Check sheet for the modelled part. Datum: model origin and axes. Units: mm. Coordinates: 2 decimals unless noted, no trailing zeros. Loops run counter-clockwise (first coordinate to the right, second up) from the corner with the lowest first, then second, coordinate; pieces in that order, holes last. Notation, with made-up numbers: (-29.5, -35.5) - (26.5, -35.5) arc R33 cw to (26.5, -3.5) - close; hole circle Ø11 at (-17.5, 81). An arc over 180 degrees is marked (long way). Write each question's results on one line, items separated by ' | '. Start each with the question number.
1. Gauge pin test, flat end, axial feed: P1, Ø1, axis at x = -3, z = 1.5, coming from the +Y side. Record the tip position at first contact, or that the pin passes through.
2. Cross-section at A-A (x = 21). Record the cut outline in (y, z).
3. Cross-section at B-B (y = 1). Record the cut outline in (x, z), and give its area (4 significant figures).
4. Cross-section at C-C (z = 1.85). Record the cut outline in (x, y).
5. Cross-section at D-D (x = -19). Record the cut outline in (y, z).
6. Draft check along Y on faces 1 (the face through (0.28, -22.22, 1.27)), 2 (the face through (24.05, -20.26, 1.27)), 3 (the face through (29, -19, 1)), 4 (the face through (10, 10, 1)). Enter one of: released by +Y, released by -Y, zero draft, split by the parting line, or undercut.
7. Thickness scan on line 1 (Y direction, x = -19, z = 1.3); line 2 (X direction, y = -20.5, z = 1.35); line 3 (Y direction, x = -22, z = 0.1). Record the ranges inside material, lowest first. Write a range as [from, to].
```python
from build123d import *

# Parameters (mm, degrees)
BOSS_EXTRUDE1_DEPTH = 2.5
SKETCH2_R           = 3.3
CUT_EXTRUDE1_DEPTH  = 3.5
LPATTERN1_COUNT     = 3
LPATTERN1_PITCH     = 20
LPATTERN2_COUNT     = 3
LPATTERN2_PITCH     = 20


with BuildPart() as part:
    # Sketch1 → Boss-Extrude1 (new body)
    with BuildSketch(Plane.XY):
        Polygon((-9, 29), (29, -9), (29, -29), (-29, -29), (-29, 29), align=None)
    extrude(amount=BOSS_EXTRUDE1_DEPTH)

    # Sketch2 → Cut-Extrude1 (cut, through all)
    with BuildSketch(Plane.XY.offset(2.5)):
        with Locations((-19, -19)):
            Circle(SKETCH2_R)
    cut_extrude1 = extrude(amount=-CUT_EXTRUDE1_DEPTH, mode=Mode.SUBTRACT)

    # LPattern1: Cut-Extrude1 ×3
    with Locations(*[(i * LPATTERN1_PITCH, 0, 0) for i in range(1, LPATTERN1_COUNT)]):
        add(cut_extrude1, mode=Mode.SUBTRACT)

    # LPattern2: Cut-Extrude1 ×3
    with Locations(*[(0, i * LPATTERN2_PITCH, 0) for i in range(1, LPATTERN2_COUNT)]):
        add(cut_extrude1, mode=Mode.SUBTRACT)


solid = part.part
```
Established:
1) P1: y = 23.5
2) outline: (-29, 0) - (-22.3, 0) - (-22.3, 2.5) - (-29, 2.5) - close; (-15.7, 0) - (-1, 0) - (-1, 2.5) - (-15.7, 2.5) - close
3) outline: (-29, 0) - (-22.3, 0) - (-22.3, 2.5) - (-29, 2.5) - close; (-15.7, 0) - (19, 0) - (19, 2.5) - (-15.7, 2.5) - close | area: 103.5 mm^2
4) outline: (-29, -29) - (29, -29) - (29, -9) - (-9, 29) - (-29, 29) - close; hole circle Ø6.6 at (-19, -19); hole circle Ø6.6 at (-19, 1); hole circle Ø6.6 at (-19, 21); hole circle Ø6.6 at (1, -19); hole circle Ø6.6 at (21, -19)
5) outline: (-29, 0) - (-22.3, 0) - (-22.3, 2.5) - (-29, 2.5) - close; (-15.7, 0) - (-2.3, 0) - (-2.3, 2.5) - (-15.7, 2.5) - close; (4.3, 0) - (17.7, 0) - (17.7, 2.5) - (4.3, 2.5) - close; (24.3, 0) - (29, 0) - (29, 2.5) - (24.3, 2.5) - close
6) face 1: undercut | face 2: undercut | face 3: zero draft | face 4: released by +Y
7) line 1: [-29, -22.3], [-15.7, -2.3], [4.3, 17.7], [24.3, 29] | line 2: [-29, -21.94], [-16.06, -1.94], [3.94, 18.06], [23.94, 29] | line 3: [-29, -20.37], [-17.63, -0.37], [2.37, 19.63], [22.37, 29]
